For this review, take the finished solid that the model builds, in its own axes (mm). Face numbers are marked on the shaded views. Coordinates: 2 decimals unless noted, no trailing zeros. Loops run counter-clockwise (first coordinate to the right, second up) from the corner with the lowest first, then second, coordinate; pieces in that order, holes last. Notation, with made-up numbers: M 70,81 L 99,81 A30 cw 99,103 Z; hole C -20.75,71 d10. An arc over 180 degrees is marked long. Use one line per item in the form item = value.
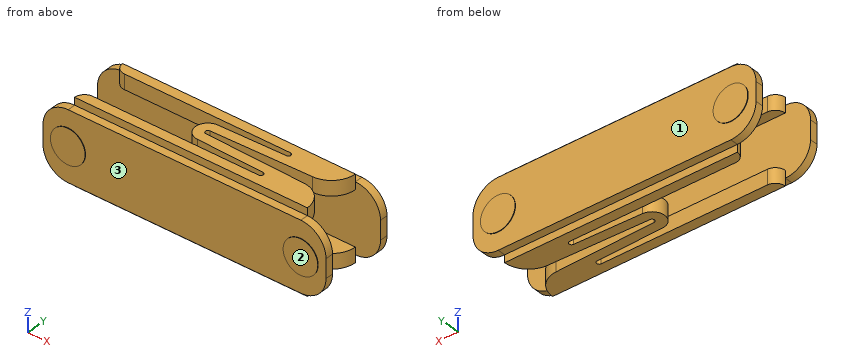
```python
from build123d import *

# Parameters (mm, degrees)
SKETCH1_W             = 57.15
SKETCH1_H             = 1.6
BOSS_EXTRUDE1_DEPTH   = 13.97
BOSS_EXTRUDE1_2_DEPTH = 13.97
FILLET1_R             = 5.08
FILLET2_R             = 5.08
BOSS_EXTRUDE3_DEPTH   = 1.5
SKETCH3_R             = 3.5
BOSS_EXTRUDE4_DEPTH   = 0.1


with BuildPart() as part:
    # Sketch1 → Boss-Extrude1 (new body)
    with BuildSketch(Plane.XY):
        with Locations((-28.575, 0.8)):
            Rectangle(SKETCH1_W, SKETCH1_H)
    extrude(amount=BOSS_EXTRUDE1_DEPTH)

    # Fillet2
    fillet2_edges = [part.edges().sort_by_distance(p)[0] for p in [
        (-57.15, 0.8, 13.97),
        (0, 0.8, 13.97),
        (-57.15, 0.8, 0),
        (0, 0.8, 0),
    ]]
    fillet(fillet2_edges, radius=FILLET2_R)



with BuildPart() as body_2:
    # Sketch1 → Boss-Extrude1 2 (new body)
    with BuildSketch(Plane.XY):
        with Locations((-28.575, 14.2)):
            Rectangle(SKETCH1_W, SKETCH1_H)
    extrude(amount=BOSS_EXTRUDE1_2_DEPTH)

    # Fillet1
    fillet1_edges = [body_2.edges().sort_by_distance(p)[0] for p in [
        (-57.15, 14.2, 13.97),
        (0, 14.2, 13.97),
        (-57.15, 14.2, 0),
        (0, 14.2, 0),
    ]]
    fillet(fillet1_edges, radius=FILLET1_R)


with BuildPart() as part_1:
    add(part.part)

    add(body_2.part)  # Boss-Extrude3 merges body 2
    # Sketch2 → Boss-Extrude3 (add, symmetric)
    with BuildSketch(Plane.XY.offset(13.97)):
        with BuildLine():
            Line((-30.014795616, 7.999781042), (-9.740002775, 8.6))
            ThreePointArc((-9.740002775, 8.6), (-6.43662966, 10.055017718), (-5.08, 13.4))
            Line((-5.08, 13.4), (-52.07, 13.4))
            ThreePointArc((-52.07, 13.4), (-51.484213562, 11.985786438), (-50.07, 11.4))
            Line((-50.07, 11.4), (-16.532798801, 11.4))
            ThreePointArc((-16.532798801, 11.4), (-16.032853544, 10.907398618), (-16.518003185, 10.400218958))
            Line((-16.518003185, 10.400218958), (-30.073978082, 9.998905209))
            ThreePointArc((-30.073978082, 9.998905209), (-32.5, 7.5), (-30.073978082, 5.001094791))
            Line((-30.073978082, 5.001094791), (-16.518003185, 4.599781042))
            ThreePointArc((-16.518003185, 4.599781042), (-16.032853544, 4.092601382), (-16.532798801, 3.6))
            Line((-16.532798801, 3.6), (-50.07, 3.6))
            ThreePointArc((-50.07, 3.6), (-51.484213562, 3.014213562), (-52.07, 1.6))
            Line((-52.07, 1.6), (-5.08, 1.6))
            ThreePointArc((-5.08, 1.6), (-6.43662966, 4.944982282), (-9.740002775, 6.4))
            Line((-9.740002775, 6.4), (-30.014795616, 7.000218958))
            ThreePointArc((-30.014795616, 7.000218958), (-30.5, 7.5), (-30.014795616, 7.999781042))
        make_face()
    boss_extrude3 = extrude(amount=BOSS_EXTRUDE3_DEPTH, both=True)

    # Mirror2: Boss-Extrude3 across plane
    add(boss_extrude3.mirror(Plane(origin=(0, 0, 6.985), x_dir=(1, 0, 0), z_dir=(0, 0, -1))))

    # Sketch3 → Boss-Extrude4 (add)
    with BuildSketch(Plane(origin=(0, 15, 0), x_dir=(1, 0, 0), z_dir=(0, 1, 0))):
        with Locations((-5.08, -6.985)):
            Circle(SKETCH3_R)
        with Locations((-52.07, -6.985)):
            Circle(SKETCH3_R)
    boss_extrude4 = extrude(amount=BOSS_EXTRUDE4_DEPTH)

    # Mirror3: Boss-Extrude4 across plane
    add(boss_extrude4.mirror(Plane.ZX.offset(7.5)))


solid = part_1.part
```
1. Wall thickness on line 1 along Y through (x, z) = (-35, 11.25); line 2 along Z through (x, y) = (-31, 7.75); line 3 along Y through (x, z) = (-2.5, 9.25): over which ranges is each line inside the solid? List them lowest first. Write a range as from..to.
Computed values:
line_1 = 0..1.6, 13.4..15
line_2 = -1.5..1.5, 12.47..15.47
line_3 = -0.1..1.6, 13.4..15.1
2. Consider section C-C on z = 4. Write out the cut boundary in (x, y), plus the area to 3 significant figures.
Computed values:
outline = M -57.03,0 L -53.9,0 L -53.9,-0.1 L -50.24,-0.1 L -50.24,0 L -6.91,0 L -6.91,-0.1 L -3.25,-0.1 L -3.25,0 L -0.12,0 L -0.12,1.6 L -57.03,1.6 Z; M -57.03,13.4 L -0.12,13.4 L -0.12,15 L -3.25,15 L -3.25,15.1 L -6.91,15.1 L -6.91,15 L -50.24,15 L -50.24,15.1 L -53.9,15.1 L -53.9,15 L -57.03,15 Z
area = 184 mm2
3. Draft analysis for pull direction X (two halves, no side actions). For the marked faces 1, 2 and 3, state which applies: +X half, -X half, draft (parallel to the pull), parting line (faces both ways), or undercut.
Computed values:
face_1 = undercut
face_2 = draft
face_3 = undercut
4. Consider section D-D on y = 1. Write out the cut boundary in (x, z).
Computed values:
outline = M -57.15,5.08 A5.08 ccw -52.07,0 L -5.08,0 A5.08 ccw 0,5.08 L 0,8.89 A5.08 ccw -5.08,13.97 L -52.07,13.97 A5.08 ccw -57.15,8.89 Z
5. For pin 1 Ø0.5 at (x, y) = (-21, 14) entering from +Z; pin 2 Ø2.5 at (x, z) = (-40, 13.5) entering from -Y; pin 3 Ø0.5 at (x, y) = (-36, 1) entering from -Z; pin 4 Ø1.5 at (y, z) = (3.5, 3.5) entering from -X, all flat-tipped, find the tip position at first contact; note any pin that passes through.
Computed values:
pin_1 = 13.97
pin_2 = 0
pin_3 = 0
pin_4 = through
6. Consider section A-A on y = 7.5. Write out the cut boundary in (x, z), plus the area to 3 significant figures.
Computed values:
outline = M -32.5,-1.5 L -30.5,-1.5 L -30.5,1.5 L -32.5,1.5 Z; M -32.5,12.47 L -30.5,12.47 L -30.5,15.47 L -32.5,15.47 Z
area = 12.0 mm2
7. Consider section B-B on x = -39. Write out the cut boundary in (y, z).
Computed values:
outline = M 0,0 L 1.6,0 L 1.6,-1.5 L 3.6,-1.5 L 3.6,1.5 L 1.6,1.5 L 1.6,12.47 L 3.6,12.47 L 3.6,15.47 L 1.6,15.47 L 1.6,13.97 L 0,13.97 Z; M 11.4,-1.5 L 13.4,-1.5 L 13.4,0 L 15,0 L 15,13.97 L 13.4,13.97 L 13.4,15.47 L 11.4,15.47 L 11.4,12.47 L 13.4,12.47 L 13.4,1.5 L 11.4,1.5 Z
